Job drawing, mm, ordinate dimensions from the low corner. One solid piece. A direction names the side the tool comes from. Coordinates: 2 decimals unless noted, no trailing zeros. Order: outer loops, then holes, each group sorted by start corner. A loop starts at its lowest first (then second) coordinate and runs counter-clockwise, first axis right, second up. Notation, with made-up numbers: (5, 49) -> (47, 49) arc R10 cw to (47, 65) -> close; hole circle Ø7 at (-5, -35). An arc over 180 degrees is marked (long way). Use CSV: the item, a comma, the result in double quotes. Start each with the question number.
(1) Cut at C-C on z = 12. Write the cut outline in (x, y), plus the area to 3 significant figures.
(2) Tool access for the marked faces 1 and 2: list every direction of +Z, -Z, +X, -X, +Y, -Y with a clear straight run to the whole face (end or side of a thin tool).
(3) Cut at B-B on y = 22.5. Write the cut outline in (x, z).
(4) Cut at A-A on x = 27.5. Write the cut outline in (y, z), plus the area to 3 significant figures.
(5) Probe L1, parallel to Y at x = 45.5, z = 67; L2, parallel to X at y = 31, z = 26. List the from-to ranges inside material, lowest first.
(6) Pull direction X, two halves, no side cores. Call the marked faces 3, 4, 5 and 6: pulls with the +X half, pulls with the -X half, needs draft (parallel to the pull), parting line crosses it, or undercut.
(7) Pin check, flat tip, straight feed: pin 1 Ø5 at (y, z) = (29, 12.5) entering from -X. Stop position of the tip, or through.
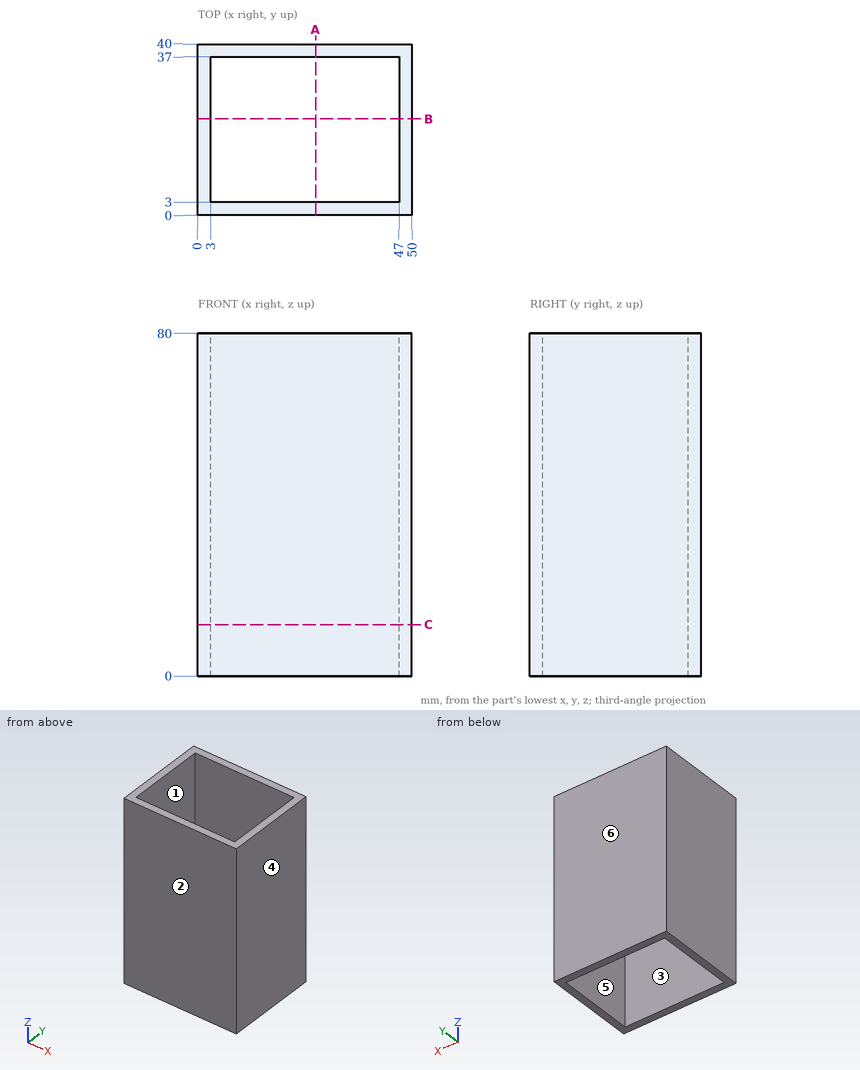
Outcome:
1,outline,"(0, 0) -> (50, 0) -> (50, 40) -> (0, 40) -> close; hole (3, 3) -> (47, 3) -> (47, 37) -> (3, 37) -> close"
1,area,"504 mm2"
2,face 1,"+Z, -Z"
2,face 2,"+Z, -Z, +X, -X, -Y"
3,outline,"(0, 0) -> (3, 0) -> (3, 80) -> (0, 80) -> close; (47, 0) -> (50, 0) -> (50, 80) -> (47, 80) -> close"
4,outline,"(0, 0) -> (3, 0) -> (3, 80) -> (0, 80) -> close; (37, 0) -> (40, 0) -> (40, 80) -> (37, 80) -> close"
4,area,"480 mm2"
5,L1,"0 to 3, 37 to 40"
5,L2,"0 to 3, 47 to 50"
6,face 3,"undercut"
6,face 4,"pulls with the +X half"
6,face 5,"undercut"
6,face 6,"needs draft"
7,pin 1,"x = 0"
